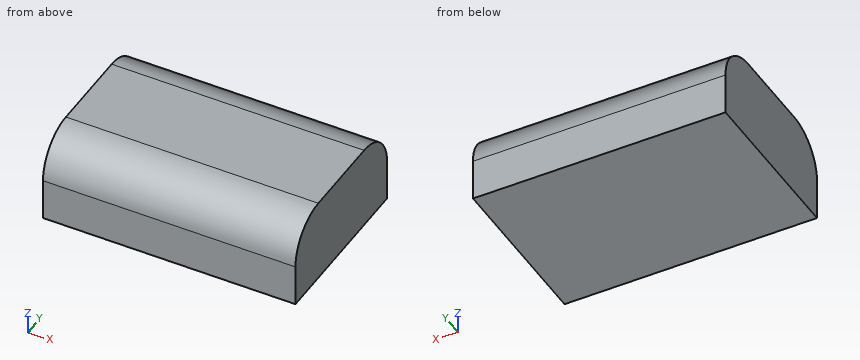
Autodesk Inventor part; units mm, degrees
ref_plane "YZ Plane" through (0, 0, 0) normal (1, 0, 0) x (0, 1, 0)
ref_plane "XZ Plane" through (0, 0, 0) normal (0, 1, 0) x (-1, 0, 0)
ref_plane "XY Plane" through (0, 0, 0) normal (0, 0, 1) x (1, 0, 0)
sketch "Эскиз1" plane through (0, 0, 0) normal (0, 0, 1) x (1, 0, 0)
  line L0 (5.2271, -13.5) -> (34.3271, -13.5)
  line L1 (15.7271, 7.05) -> (6.6989, 7.05)
  line L2 (-4.4915, 7.05) -> (-34.4915, 7.05)
  line L3 (-34.4915, 7.05) -> (-34.4915, -12.95)
  line L4 (-34.4915, -12.95) -> (-4.4915, -12.95)
  line L5 (-4.4915, -12.95) -> (-4.4915, 7.05)
  point P0 (0, 0)
  dimension "d0" = 20
  dimension "d2" = 30
extrude "Выдавливание1" add sketch "Эскиз1" along normal blind 10
fillet "Сопряжение1" radius 5 2 edges at (-19.4915, -12.95, 10) (-19.4915, 7.05, 10)
properties part number "Интвертор"
Part model, mm, in its own coordinate system. Round coordinates to 2 decimals unless told otherwise and drop trailing zeros. Loops run counter-clockwise (first coordinate to the right, second up) from the corner with the lowest first, then second, coordinate; pieces in that order, holes last. Notation, with made-up numbers: (-31.75, 42.25) -> (0.25, 42.25) arc R21 cw to (0.25, 54.25) -> close; hole circle Ø3 at (5, 72). An arc over 180 degrees is marked (long way). Use one line per item in the form item = value. Start each with the question number.
Item 1: Drill centre lines: line 1 along Y through (x, z) = (-6.25, 5.25); line 2 along Y through (x, z) = (-28.5, 9.5); line 3 along Z through (x, y) = (-16.75, 4). Where is each one in solid material? Low to high.
Item 2: Drop a flat-ended pin along its axis: pin 1 Ø2 at (x, z) = (-15, 6.5) entering from +Y. Give the stop position or say it passes through.
Item 3: Band-saw the part on A-A (x = -11). List the corners of the cut face in (y, z).
Item 4: Band-saw the part on C-C (y = 4.75). List the corners of the cut face in (x, z), plus the area to 3 significant figures.
Item 5: Band-saw the part on B-B (z = 9). List the corners of the cut face in (x, y), plus the area to 3 significant figures.
Data:
q1.line_1 = -12.94 to 7.04
q1.line_2 = -10.13 to 4.23
q1.line_3 = 0 to 9.6
q2.pin_1 = 7.02
q3.outline = (-12.95, 0) -> (7.05, 0) -> (7.05, 5) arc R5 ccw to (2.05, 10) -> (-7.95, 10) arc R5 ccw to (-12.95, 5) -> close
q4.outline = (-34.49, 0) -> (-4.49, 0) -> (-4.49, 9.21) -> (-34.49, 9.21) -> close
q4.area = 276 mm^2
q5.outline = (-34.49, -10.95) -> (-4.49, -10.95) -> (-4.49, 5.05) -> (-34.49, 5.05) -> close
q5.area = 480 mm^2
